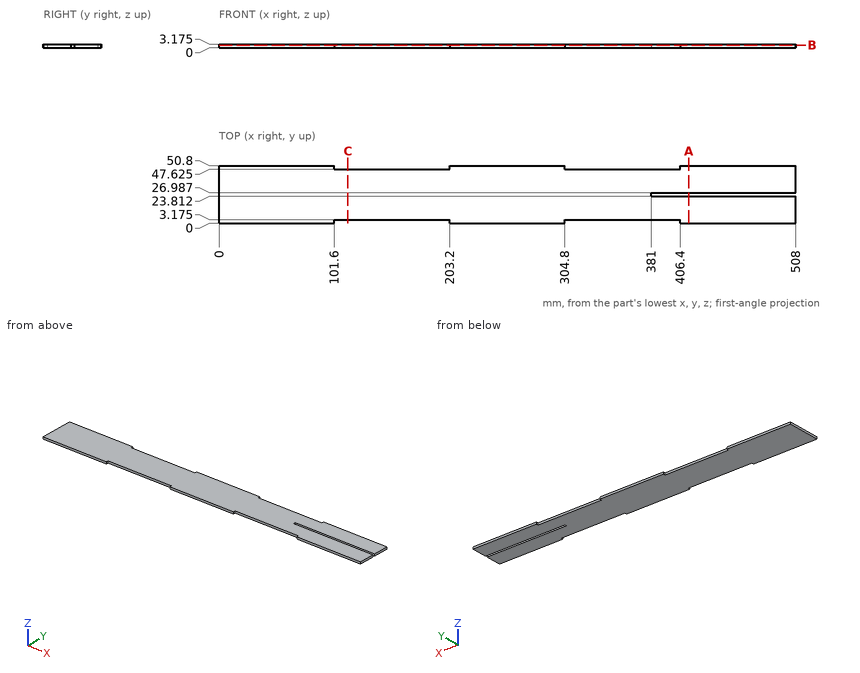
Source: three-view drawing plus pictorial views. Frame: mm from the lowest corner of the part. Coordinates: 2 decimals unless noted, no trailing zeros. Loops run counter-clockwise (first coordinate to the right, second up) from the corner with the lowest first, then second, coordinate; pieces in that order, holes last. Notation, with made-up numbers: (13, 25) -> (29, 25) arc R23 cw to (29, 34) -> close; hole circle Ø10 at (-1, -35.75). An arc over 180 degrees is marked (long way). Write each question's results on one line, items separated by ' | '. Start each with the question number.
Q1. Section C-C, the plane x = 113.5. Return the cut outline in (y, z) (1 decimal), plus the area to 3 significant figures.
Q2. Section A-A, the plane x = 414. Return the cut outline in (y, z) (1 decimal).
Q3. Section B-B, the plane z = 2.1. Return the cut outline in (x, y) (1 decimal).
Q4. Pin query (flat end, axial travel): pin 1 (1.6 mm diameter, centred on x = 470, z = 2, fed in from -Y); pin 2 (1.6 mm diameter, centred on x = 372, z = 1, fed in from +Y) (1 decimal). Return the tip coordinate at first contact, or that it passes through.
Q5. Ray query, line 1 (Y direction, x = 449, z = 0.35); line 2 (Y direction, x = 114, z = 2.5) (1 decimal); line 3 (Y direction, x = 381.5, z = 2.75) (1 decimal). Return the intervals inside material, ascending. Write a range as from..to.
Found:
1) outline: (3.2, 0) -> (47.6, 0) -> (47.6, 3.2) -> (3.2, 3.2) -> close | area: 141 mm2
2) outline: (0, 0) -> (23.8, 0) -> (23.8, 3.2) -> (0, 3.2) -> close; (27, 0) -> (50.8, 0) -> (50.8, 3.2) -> (27, 3.2) -> close
3) outline: (0, 0) -> (101.6, 0) -> (101.6, 3.2) -> (203.2, 3.2) -> (203.2, 0) -> (304.8, 0) -> (304.8, 3.2) -> (406.4, 3.2) -> (406.4, 0) -> (508, 0) -> (508, 23.8) -> (381, 23.8) -> (381, 27) -> (508, 27) -> (508, 50.8) -> (406.4, 50.8) -> (406.4, 47.6) -> (304.8, 47.6) -> (304.8, 50.8) -> (203.2, 50.8) -> (203.2, 47.6) -> (101.6, 47.6) -> (101.6, 50.8) -> (0, 50.8) -> close
4) pin 1: y = 0 | pin 2: y = 47.6
5) line 1: 0..23.81, 26.99..50.8 | line 2: 3.2..47.6 | line 3: 3.2..23.8, 27..47.6
